Build history of the part. All positions in model axes, mm. Give positions to 0.01 mm unless a question says otherwise; leave off trailing zeros. Write each loop counter-clockwise with the first axis right and the second up, starting at its lowest first coordinate (ties: lowest second). Pieces come first, ordered by that corner, then holes. Notation, with made-up numbers: (17.5, -16) -> (26.5, -16) arc R10 ccw to (26.5, -10) -> close; hole circle Ø8 at (85.5, 68). An arc over 180 degrees is marked (long way). Put each result on its own line as item: value. Start each with the question number.
Item 1: Flat gauge pins, fed straight in: pin 1 Ø1.2 at (y, z) = (3.5, -29) entering from -X; pin 2 Ø2.5 at (x, y) = (27.5, 3) entering from +Z; pin 3 Ø1.2 at (y, z) = (3.5, -24) entering from +X; pin 4 Ø0.6 at (x, y) = (1, 3) entering from -Z. Where does each tip first touch, or does it go through?
Item 2: Drill centre lines: line 1 along X through (y, z) = (2.55, -27.5); line 2 along Z through (x, y) = (49, 2); line 3 along X through (y, z) = (2, -47.5). Where is each one in solid material? Low to high.
Item 3: Slice it at A-A, the plane x = 39. List the corners of the cut face in (y, z), plus the area to 3 significant figures.
Item 4: Slice it at B-B, the plane y = 3.65. List the corners of the cut face in (x, z), plus the area to 3 significant figures.
Item 5: Slice it at C-C, the plane z = -41.5. List the corners of the cut face in (x, y), plus the area to 3 significant figures.
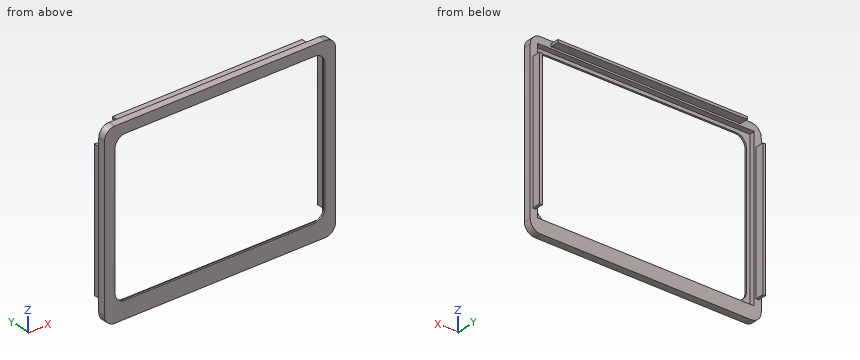
```python
from build123d import *

# Parameters (mm, degrees)
BOSS_EXTRUDE1_DEPTH = 2.1
SKETCH3_W           = 63
SKETCH3_H           = 46
CUT_EXTRUDE1_DEPTH  = 1.6
CUT_EXTRUDE2_DEPTH  = 0.5
SKETCH6_W           = 0.75
SKETCH6_H           = 40
SKETCH6_W_2         = 55
SKETCH6_H_2         = 0.75
BOSS_EXTRUDE2_DEPTH = 2.5


with BuildPart() as part:
    # Sketch1 → Boss-Extrude1 (new body)
    with BuildSketch(Plane(origin=(0, 0, 0), x_dir=(1, 0, 0), z_dir=(0, 1, 0))):
        with BuildLine():
            Line((3, 0), (64.1, 0))
            ThreePointArc((64.1, 0), (66.221320344, 0.878679656), (67.1, 3))
            Line((67.1, 3), (67.1, 49))
            ThreePointArc((67.1, 49), (66.221320344, 51.121320344), (64.1, 52))
            Line((64.1, 52), (3, 52))
            ThreePointArc((3, 52), (0.878679656, 51.121320344), (0, 49))
            Line((0, 49), (0, 3))
            ThreePointArc((0, 3), (0.878679656, 0.878679656), (3, 0))
        make_face()
    extrude(amount=BOSS_EXTRUDE1_DEPTH)

    # Sketch3 → Cut-Extrude1 (cut)
    with BuildSketch(Plane(origin=(0, 2.1, 0), x_dir=(1, 0, 0), z_dir=(0, 1, 0))):
        with Locations((33.55, 25.05)):
            Rectangle(SKETCH3_W, SKETCH3_H)
    extrude(amount=-CUT_EXTRUDE1_DEPTH, mode=Mode.SUBTRACT)

    # Sketch5 → Cut-Extrude2 (cut)
    with BuildSketch(Plane(origin=(0, 0.5, 0), x_dir=(1, 0, 0), z_dir=(0, 1, 0))):
        with BuildLine():
            Line((6.05, 47.05), (61.05, 47.05))
            ThreePointArc((61.05, 47.05), (63.171320344, 46.171320344), (64.05, 44.05))
            Line((64.05, 44.05), (64.05, 6.05))
            ThreePointArc((64.05, 6.05), (63.171320344, 3.928679656), (61.05, 3.05))
            Line((61.05, 3.05), (6.05, 3.05))
            ThreePointArc((6.05, 3.05), (3.928679656, 3.928679656), (3.05, 6.05))
            Line((3.05, 6.05), (3.05, 44.05))
            ThreePointArc((3.05, 44.05), (3.928679656, 46.171320344), (6.05, 47.05))
        make_face()
    extrude(amount=-CUT_EXTRUDE2_DEPTH, mode=Mode.SUBTRACT)

    # Sketch6 → Boss-Extrude2 (add)
    with BuildSketch(Plane(origin=(0, 2.1, 0), x_dir=(1, 0, 0), z_dir=(0, 1, 0))):
        with Locations((65.975, 26)):
            Rectangle(SKETCH6_W, SKETCH6_H)
        with Locations((1.125, 26)):
            Rectangle(SKETCH6_W, SKETCH6_H)
        with Locations((33.55, 1.125)):
            Rectangle(SKETCH6_W_2, SKETCH6_H_2)
    extrude(amount=BOSS_EXTRUDE2_DEPTH)


solid = part.part
```
Values follow:
1. pin 1: x = 0.75
1. pin 2: z = 0
1. pin 3: x = 66.35
1. pin 4: z = -46
2. line 1: 0.75 to 1.5, 65.6 to 66.35
2. line 2: -52 to -48.05, -2.05 to 0
2. line 3: 0 to 2.05, 65.05 to 67.1
3. outline: (0, -52) -> (2.1, -52) -> (2.1, -48.05) -> (0.5, -48.05) -> (0.5, -47.05) -> (0, -47.05) -> close; (0, -3.05) -> (0.5, -3.05) -> (0.5, -2.05) -> (2.1, -2.05) -> (2.1, -1.5) -> (4.6, -1.5) -> (4.6, -0.75) -> (2.1, -0.75) -> (2.1, 0) -> (0, 0) -> close
3. area: 15.5 mm2
4. outline: (0.75, -46) -> (1.5, -46) -> (1.5, -6) -> (0.75, -6) -> close; (6.05, -1.5) -> (61.05, -1.5) -> (61.05, -0.75) -> (6.05, -0.75) -> close; (65.6, -46) -> (66.35, -46) -> (66.35, -6) -> (65.6, -6) -> close
4. area: 101 mm2
5. outline: (0, 0) -> (3.05, 0) -> (3.05, 0.5) -> (2.05, 0.5) -> (2.05, 2.1) -> (1.5, 2.1) -> (1.5, 4.6) -> (0.75, 4.6) -> (0.75, 2.1) -> (0, 2.1) -> close; (64.05, 0) -> (67.1, 0) -> (67.1, 2.1) -> (66.35, 2.1) -> (66.35, 4.6) -> (65.6, 4.6) -> (65.6, 2.1) -> (65.05, 2.1) -> (65.05, 0.5) -> (64.05, 0.5) -> close
5. area: 13.4 mm2
